Here's the drawing with two shaded views (mm, measured from the low corner). I have some questions. A direction names the side the tool comes from. Coordinates: 2 decimals unless noted, no trailing zeros. Order: outer loops, then holes, each group sorted by start corner. A loop starts at its lowest first (then second) coordinate and runs counter-clockwise, first axis right, second up. Notation, with made-up numbers: (84.25, -28) - (143.25, -28) arc R20 cw to (143.25, 10) - close; hole circle Ø9 at (49.25, -24.5). An arc over 180 degrees is marked (long way). Answer as a JSON object with one key per item and string values. Group by question number.
(1) We'd pull the mould along Y, two halves only. Please class the marked faces 1, 2 and 3: pulls with the +Y half, pulls with the -Y half, needs draft (parallel to the pull), parting line crosses it, or undercut.
(2) Which directions (+Z, -Z, +X, -X, +Y, -Y) give clear straight access to the entire face, cutting with the end or side of a thin tool? Please do the marked faces 4 and 5.
(3) Imagine slicing it at B-B, the plane x = 7.5. Write out the boundary of the cut face in (y, z), and give its area (3 significant figures).
(4) Please list where these lines run through material, in increasing order: probe 1 along Y at (x, z) = (5.5, 1.4); probe 2 along X at (y, z) = (14.5, 1.8); probe 3 along Y at (x, z) = (8, 0.6).
(5) Imagine slicing it at D-D, the plane x = 4.5. Write out the boundary of the cut face in (y, z), and give its area (3 significant figures).
(6) Will this pin go through, and if not, where does the flat tip stop? P1, Ø1.6, axis at x = 5, z = 2, coming from the -Y side.
(7) Imagine slicing it at A-A, the plane y = 21.5. Write out the boundary of the cut face in (x, z), and give its area (3 significant figures).
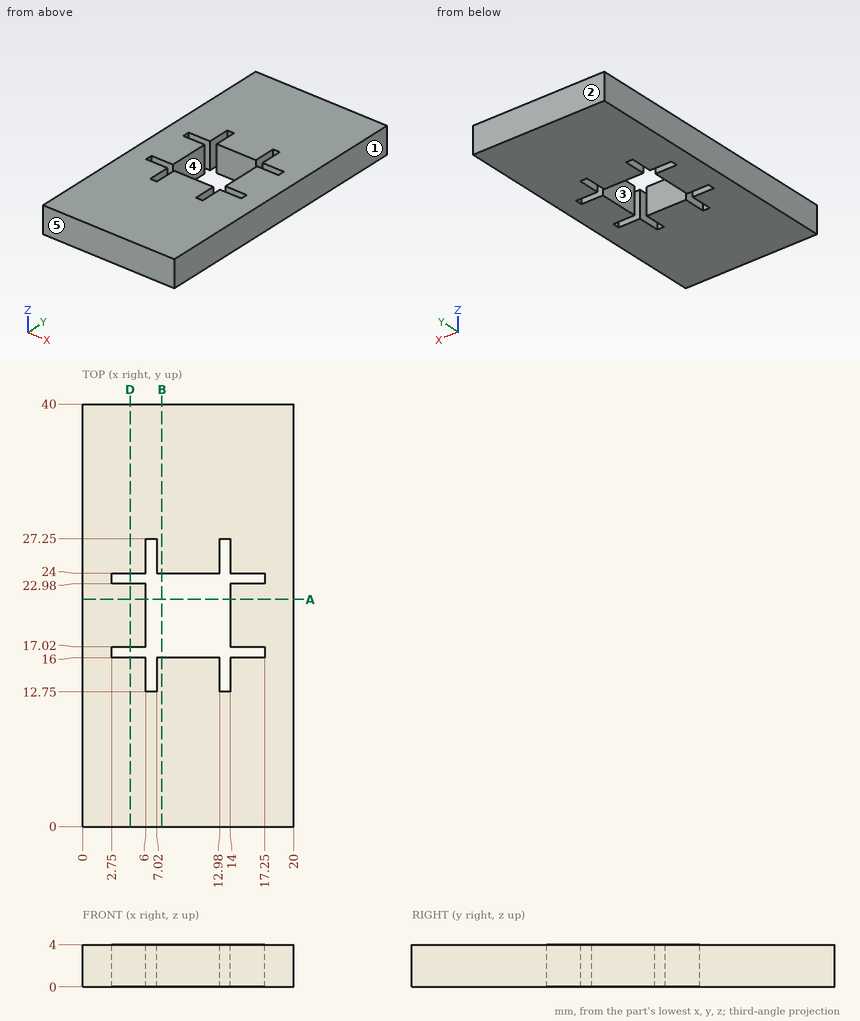
Result set:
{
 "1": {"face 1": "needs draft", "face 2": "pulls with the +Y half", "face 3": "undercut"},
 "2": {"face 4": "+Z, -Z", "face 5": "+Z, -Z, +X, -X, -Y"},
 "3": {"outline": "(0, 0) - (16, 0) - (16, 4) - (0, 4) - close; (24, 0) - (40, 0) - (40, 4) - (24, 4) - close", "area": "128 mm^2"},
 "4": {"probe 1": "y = 0 to 16, 17.02 to 22.98, 24 to 40", "probe 2": "x = 0 to 6, 7.02 to 12.98, 14 to 20", "probe 3": "y = 0 to 16, 24 to 40"},
 "5": {"outline": "(0, 0) - (16, 0) - (16, 4) - (0, 4) - close; (17.02, 0) - (22.98, 0) - (22.98, 4) - (17.02, 4) - close; (24, 0) - (40, 0) - (40, 4) - (24, 4) - close", "area": "152 mm^2"},
 "6": {"P1": "stops at y = 0"},
 "7": {"outline": "(0, 0) - (6, 0) - (6, 4) - (0, 4) - close; (14, 0) - (20, 0) - (20, 4) - (14, 4) - close", "area": "48.0 mm^2"}
}
